Verification items for the finished model (mm, model axes). A direction names the side the tool comes from. Round coordinates to 2 decimals unless told otherwise and drop trailing zeros. Order: outer loops, then holes, each group sorted by start corner. A loop starts at its lowest first (then second) coordinate and runs counter-clockwise, first axis right, second up.
```python
from build123d import *

# Parameters (mm, degrees)
BOSS_EXTRUDE1_DEPTH = 16
FILLET3_R           = 0.8
CUT_EXTRUDE1_START  = 5
SKETCH3_R           = 11.65
CUT_EXTRUDE1_DEPTH  = 33
SKETCH2_R           = 3.1
BOSS_EXTRUDE2_DEPTH = 5
BOSS_EXTRUDE2_TAPER = 5
CUT_EXTRUDE2_DEPTH  = 67.627997142
FILLET1_R           = 5
FILLET2_R           = 1
CHAMFER2_SIZE       = 0.8


with BuildPart() as part:
    # Sketch1 → Boss-Extrude1 (new body)
    with BuildSketch(Plane.XY):
        Polygon((0, 0), (0, 57.3), (5, 57.3), (5, 5), (25, 5), (25, 57.3), (30, 57.3), (30, 0), align=None)
    extrude(amount=BOSS_EXTRUDE1_DEPTH)

    # Fillet3
    fillet3_edges = [part.edges().sort_by_distance(p)[0] for p in [
        (5, 5, 8),
        (25, 5, 8),
    ]]
    fillet(fillet3_edges, radius=FILLET3_R)

    # Sketch3 → Cut-Extrude1 (cut)
    with BuildSketch(Plane(origin=(0, 0, 0), x_dir=(1, 0, 0), z_dir=(0, 1, 0)).offset(CUT_EXTRUDE1_START)):
        with Locations((15, -8)):
            Circle(SKETCH3_R)
    extrude(amount=CUT_EXTRUDE1_DEPTH, mode=Mode.SUBTRACT)

    # Sketch2 → Boss-Extrude2 (add)
    with BuildSketch(Plane(origin=(0, 5, 0), x_dir=(1, 0, 0), z_dir=(0, 1, 0))):
        with Locations((15, -8)):
            Circle(SKETCH2_R)
    extrude(amount=BOSS_EXTRUDE2_DEPTH, taper=BOSS_EXTRUDE2_TAPER)

    # Sketch5 → Cut-Extrude2 (cut, through all)
    with BuildSketch(Plane(origin=(30, 0, 0), x_dir=(0, 0, -1), z_dir=(1, 0, 0))):
        with BuildLine():
            Line((-5.4, 47.8), (-5.4, 46.8))
            ThreePointArc((-5.4, 46.8), (-8, 44.2), (-10.6, 46.8))
            Line((-10.6, 46.8), (-10.6, 47.8))
            ThreePointArc((-10.6, 47.8), (-8, 50.4), (-5.4, 47.8))
        make_face()
    extrude(amount=-CUT_EXTRUDE2_DEPTH, mode=Mode.SUBTRACT)

    # Fillet1
    fillet1_edges = [part.edges().sort_by_distance(p)[0] for p in [
        (0, 0, 8),
        (30, 0, 8),
        (30, 57.3, 8),
        (0, 57.3, 8),
    ]]
    fillet(fillet1_edges, radius=FILLET1_R - 0.0001)  # a hair under: the kernel refuses the full size

    # Fillet2
    fillet2_edges = [part.edges().sort_by_distance(p)[0] for p in [
        (5, 57.3, 8),
        (25, 57.3, 8),
        (12.337443318, 10, 8),
    ]]
    fillet(fillet2_edges, radius=FILLET2_R)

    # Chamfer2
    chamfer2_edges = [part.edges().sort_by_distance(p)[0] for p in [
        (1.047161628, 55.361939214, 0),
        (30, 28.65, 16),
        (15, 0, 16),
        (0, 28.65, 16),
        (28.535563195, 1.464436805, 16),
        (1.464436805, 1.464436805, 16),
        (28.952838372, 55.361939214, 16),
        (25, 30.986502943, 16),
        (25, 30.986502943, 0),
        (28.952838372, 55.361939214, 0),
        (4.61238009, 56.963569371, 0),
        (25.38761991, 56.963569371, 0),
        (1.047161628, 55.361939214, 16),
        (4.61238009, 56.963569371, 16),
        (25.38761991, 56.963569371, 16),
        (5, 30.986502943, 0),
        (5, 30.986502943, 16),
        (15, 5, 0),
        (15, 5, 16),
        (5.234314575, 5.234314575, 0),
        (5.234314575, 5.234314575, 16),
        (24.765685425, 5.234314575, 0),
        (24.765685425, 5.234314575, 16),
        (15, 0, 0),
        (0, 28.65, 0),
        (30, 28.65, 0),
        (28.535563195, 1.464436805, 0),
        (1.464436805, 1.464436805, 0),
    ]]
    chamfer(chamfer2_edges, length=CHAMFER2_SIZE)


solid = part.part
```
1) Sectioned sample at B-B on x = 19.5. Record the cut outline in (y, z), then the cut area to 3 significant figures.
2) Go/stop test with flat-tipped pins: pin 1 Ø0.5 at (x, z) = (4, 6.5) entering from -Y; pin 2 Ø1 at (x, z) = (15, 8.5) entering from +Y; pin 3 Ø1 at (x, z) = (16, 2.5) entering from +Y. Record where each tip stops, or that it passes through.
3) Sectioned sample at C-C on z = 8. Count the separate pieces of the cut face and the enclosed holes in it, then the cut area to 3 significant figures.
4) Sectioned sample at D-D on x = 15. Record the cut outline in (y, z).
5) Sectioned sample at A-A on y = 36. Record the cut outline in (x, z), then the cut area to 3 significant figures.
6) Scan lines: probe 1 along X at (y, z) = (36.5, 8); probe 2 along X at (y, z) = (31, 15); probe 3 along Y at (x, z) = (11, 10). Record each from-to range of solid material in increasing order.
7) Tool access check on faces 5 (the flat face through (12, 5, 6)), 6 (the cylindrical face through (27.5, 44.2, 7.9)), 7 (the flat face through (15, 10, 8)). Record the directions out of +Z, -Z, +X, -X, +Y, -Y that give a thin tool (end or side, any length) a straight path to the whole face; none if there is none.
8) Draft check along X on faces 1 (the conical face through (1.97, 1.91, 15.87)), 2 (the flat face through (5, 43, 8)), 3 (the flat face through (26, 38, 8)), 4 (the conical face through (28.034, 1.898, 0.139)). Enter one of: released by +X, released by -X, zero draft, split by the parting line, or undercut.
Returned:
1. outline: (0, 0.8) - (0.8, 0) - (4.2, 0) - (5, 0.8) - (5, 15.2) - (4.2, 16) - (0.8, 16) - (0, 15.2) - close
1. area: 78.7 mm2
2. pin 1: stops at y = 0.06
2. pin 2: stops at y = 10
2. pin 3: stops at y = 5
3. separate pieces: 3
3. enclosed holes: 0
3. area: 508 mm2
4. outline: (0, 0.8) - (0.8, 0) - (4.2, 0) - (5, 0.8) - (5, 4.9) - (9.09, 5.26) arc R1 ccw to (10, 6.25) - (10, 9.75) arc R1 ccw to (9.09, 10.74) - (5, 11.1) - (5, 15.2) - (4.2, 16) - (0.8, 16) - (0, 15.2) - close
5. outline: (0, 0.8) - (0.8, 0) - (4.2, 0) - (5, 0.8) - (5, 2.02) arc R11.65 cw to (5, 13.98) - (5, 15.2) - (4.2, 16) - (0.8, 16) - (0, 15.2) - close; (25, 0.8) - (25.8, 0) - (29.2, 0) - (30, 0.8) - (30, 15.2) - (29.2, 16) - (25.8, 16) - (25, 15.2) - (25, 13.98) arc R11.65 cw to (25, 2.02) - close
5. area: 131 mm2
6. probe 1: x = 0 to 3.35, 26.65 to 30
6. probe 2: x = 0 to 5, 25 to 30
6. probe 3: y = 0 to 5
7. face 5: none
7. face 6: +X, -X
7. face 7: +Z, -Z, +Y
8. face 1: released by -X
8. face 2: undercut
8. face 3: undercut
8. face 4: released by +X
